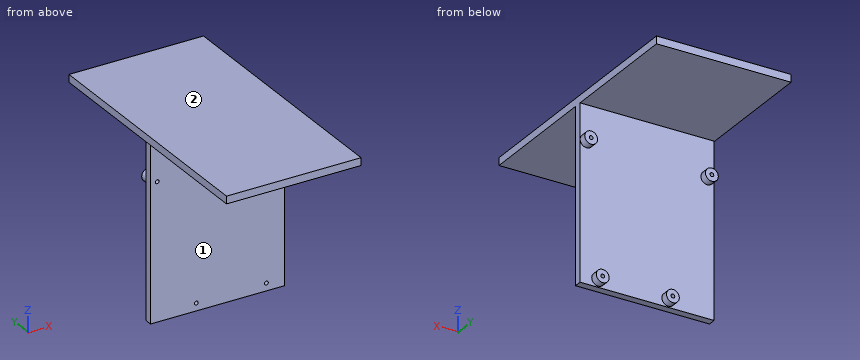
from build123d import *

# Parameters (mm, degrees)
F0_W     = 53.3
F0_H     = 72
F0_R     = 2.55
F0_R_2   = 0.75
F1_DEPTH = 3
F2_DEPTH = 3
F3_DEPTH = 3
F4_W     = 53.492
F4_H     = 3
F5_DEPTH = 53
F6_DEPTH = 50


with BuildPart() as f1:
    # F0 (on Front) → F1 (new body)
    with BuildSketch(Plane.XZ):
        with Locations((-26.65, -36)):
            Rectangle(F0_W, F0_H)
        with Locations((-35.1, -69)):
            Circle(F0_R, mode=Mode.SUBTRACT)
        with Locations((-7.2, -69)):
            Circle(F0_R, mode=Mode.SUBTRACT)
        with Locations((-50.6, -18)):
            Circle(F0_R, mode=Mode.SUBTRACT)
        with Locations((-2.6, -17)):
            Circle(F0_R, mode=Mode.SUBTRACT)
        with Locations((-50.6, -18)):
            Circle(F0_R)
        with Locations((-50.6, -18)):
            Circle(F0_R_2, mode=Mode.SUBTRACT)
        with Locations((-2.6, -17)):
            Circle(F0_R)
        with Locations((-2.6, -17)):
            Circle(F0_R_2, mode=Mode.SUBTRACT)
        with Locations((-7.2, -69)):
            Circle(F0_R)
        with Locations((-7.2, -69)):
            Circle(F0_R_2, mode=Mode.SUBTRACT)
        with Locations((-35.1, -69)):
            Circle(F0_R)
        with Locations((-35.1, -69)):
            Circle(F0_R_2, mode=Mode.SUBTRACT)
    extrude(amount=F1_DEPTH)

    # F0 (on Front) → F2 (join)
    with BuildSketch(Plane.XZ):
        with Locations((-50.6, -18)):
            Circle(F0_R)
        with Locations((-50.6, -18)):
            Circle(F0_R_2, mode=Mode.SUBTRACT)
        with Locations((-2.6, -17)):
            Circle(F0_R)
        with Locations((-2.6, -17)):
            Circle(F0_R_2, mode=Mode.SUBTRACT)
        with Locations((-7.2, -69)):
            Circle(F0_R)
        with Locations((-7.2, -69)):
            Circle(F0_R_2, mode=Mode.SUBTRACT)
        with Locations((-35.1, -69)):
            Circle(F0_R)
        with Locations((-35.1, -69)):
            Circle(F0_R_2, mode=Mode.SUBTRACT)
    extrude(amount=-F2_DEPTH)

    # F0 (on Front) → F3 (cut)
    with BuildSketch(Plane.XZ):
        with Locations((-2.6, -17)):
            Circle(F0_R_2)
        with Locations((-50.6, -18)):
            Circle(F0_R_2)
        with Locations((-35.1, -69)):
            Circle(F0_R_2)
        with Locations((-7.2, -69)):
            Circle(F0_R_2)
    extrude(amount=-F3_DEPTH, mode=Mode.SUBTRACT)

    # F4 (on Front) → F5 (join)
    with BuildSketch(Plane.XZ):
        with Locations((-26.746, -1.5)):
            Rectangle(F4_W, F4_H)
    extrude(amount=F5_DEPTH)

    # F4 (on Front) → F6 (join)
    with BuildSketch(Plane.XZ):
        with Locations((-26.746, -1.5)):
            Rectangle(F4_W, F4_H)
    extrude(amount=-F6_DEPTH)


solid = f1.part
Check sheet for the modelled part. Datum: model origin and axes. Units: mm. Face numbers are marked on the shaded views. A direction names the side the tool comes from. Round coordinates to 2 decimals unless told otherwise and drop trailing zeros. Loops run counter-clockwise (first coordinate to the right, second up) from the corner with the lowest first, then second, coordinate; pieces in that order, holes last. Notation, with made-up numbers: (63.25, -12) -> (115.25, -12) arc R25 ccw to (115.25, 14) -> close; hole circle Ø7 at (36.25, -27). An arc over 180 degrees is marked (long way). Put each result on its own line as item: value. Start each with the question number.
1. Gauge pin test, flat ends, axial feed: pin 1 (1.7 mm diameter, centred on x = -35.1, z = -69, fed in from +Y); pin 2 (2.5 mm diameter, centred on y = -2, z = -44, fed in from -X); pin 3 (1.7 mm diameter, centred on x = -7.2, z = -69, fed in from -Y). Record the tip position at first contact, or that the pin passes through.
2. Scan lines: probe 1 along X at (y, z) = (-0.1, -69); probe 2 along Z at (x, y) = (-35.1, 1.45); probe 3 along Z at (x, y) = (-2.6, 0.25). Record each from-to range of solid material in increasing order.
3. Section check B-B (y = -34). Enter the section's corners in (x, z).
4. Access from +Z, -Z, +X, -X, +Y, -Y to the whole of each face (thin tool, end or side, straight path). Record for the marked faces 1 and 2.
5. Section check C-C (z = -49). Enter the section's corners in (x, y).
6. Section check A-A (x = -41). Enter the section's corners in (y, z).
Findings:
1. pin 1: stops at y = 3
1. pin 2: stops at x = -53.3
1. pin 3: stops at y = -3
2. probe 1: x = -53.3 to -35.85, -34.35 to -7.95, -6.45 to 0
2. probe 2: z = -71.55 to -69.75, -68.25 to -66.45, -3 to 0
2. probe 3: z = -19.55 to -17.75, -16.25 to -14.45, -3 to 0
3. outline: (-53.49, -3) -> (0, -3) -> (0, 0) -> (-53.49, 0) -> close
4. face 1: -Z, +X, -X, -Y
4. face 2: +Z, +X, -X, +Y, -Y
5. outline: (-53.3, -3) -> (0, -3) -> (0, 0) -> (-53.3, 0) -> close
6. outline: (-53, -3) -> (-3, -3) -> (-3, -72) -> (0, -72) -> (0, -3) -> (50, -3) -> (50, 0) -> (-53, 0) -> close
